```python
from build123d import *

# Parameters (mm, degrees)
SKETCH041_R   = 1.6
SKETCH041_R_2 = 5.98
PAD_DEPTH     = 5


with BuildPart() as part:
    # Sketch041 → Pad (new body)
    with BuildSketch(Plane.XZ):
        with BuildLine():
            Line((75.17, -33), (80.83, -33))
            Line((80.83, -33), (88.709309, -17.413936))
            ThreePointArc((88.709309, -17.413936), (89.672868, -14.782831), (90, -12))
            Line((90, -12), (90, -4))
            ThreePointArc((90, -4), (86.485281, 4.485281), (78, 8))
            Line((78, 8), (31, 8))
            ThreePointArc((28, 11), (28.87868, 8.87868), (31, 8))
            ThreePointArc((28, 11), (27.707107, 11.707107), (27, 12))
            Line((27, 12), (-19, 12))
            ThreePointArc((-19, 12), (-19.707107, 11.707107), (-20, 11))
            Line((-20, 11), (-20, -24))
            Line((-20, -24), (72.36, -24))
            Line((72.36, -24), (75.17, -33))
        make_face()
        with Locations((-14, 7)):
            Circle(SKETCH041_R, mode=Mode.SUBTRACT)
        with Locations((-2, -18)):
            Circle(SKETCH041_R, mode=Mode.SUBTRACT)
        Circle(SKETCH041_R_2, mode=Mode.SUBTRACT)
        with Locations((78, -12)):
            Circle(SKETCH041_R_2, mode=Mode.SUBTRACT)
        with BuildLine():
            ThreePointArc((7.5, -12.2), (8.027208, -13.472792), (9.3, -14))
            Line((9.3, -14), (13.2, -14))
            ThreePointArc((13.2, -14), (14.472792, -13.472792), (15, -12.2))
            Line((15, -12.2), (15, -9.8))
            ThreePointArc((15, -9.8), (14.472792, -8.527208), (13.2, -8))
            Line((13.2, -8), (9.3, -8))
            ThreePointArc((9.3, -8), (8.027208, -8.527208), (7.5, -9.8))
            Line((7.5, -9.8), (7.5, -12.2))
        make_face(mode=Mode.SUBTRACT)
        with BuildLine():
            Line((17.7, -4.5), (24.3, -4.5))
            ThreePointArc((24.3, -4.5), (25.148528, -4.148528), (25.5, -3.3))
            Line((25.5, -3.3), (25.5, -2.7))
            ThreePointArc((25.5, -2.7), (25.148528, -1.851472), (24.3, -1.5))
            Line((24.3, -1.5), (17.7, -1.5))
            ThreePointArc((17.7, -1.5), (16.851472, -1.851472), (16.5, -2.7))
            Line((16.5, -2.7), (16.5, -3.3))
            ThreePointArc((16.5, -3.3), (16.851472, -4.148528), (17.7, -4.5))
        make_face(mode=Mode.SUBTRACT)
        with BuildLine():
            Line((17.7, -16), (24.3, -16))
            ThreePointArc((24.3, -16), (25.148528, -15.648528), (25.5, -14.8))
            Line((25.5, -14.8), (25.5, -12.2))
            ThreePointArc((25.5, -12.2), (25.148528, -11.351472), (24.3, -11))
            Line((24.3, -11), (17.7, -11))
            ThreePointArc((17.7, -11), (16.851472, -11.351472), (16.5, -12.2))
            Line((16.5, -12.2), (16.5, -14.8))
            ThreePointArc((16.5, -14.8), (16.851472, -15.648528), (17.7, -16))
        make_face(mode=Mode.SUBTRACT)
    extrude(amount=PAD_DEPTH)


solid = part.part
```
Geometry check sheet. Reference: the model listing, model coordinates, mm. A direction names the side the tool comes from. Round coordinates to 2 decimals unless told otherwise and drop trailing zeros. Order: outer loops, then holes, each group sorted by start corner. A loop starts at its lowest first (then second) coordinate and runs counter-clockwise, first axis right, second up. Notation, with made-up numbers: (51.5, -16) -> (96.5, -16) arc R16 cw to (96.5, -9) -> close; hole circle Ø11 at (39, 49.25). An arc over 180 degrees is marked (long way). Return JSON: item names as keys, results as strings. Group by question number.
Q1. Material ranges on probe 1 along Z at (x, y) = (78, -0.95); probe 2 along Z at (x, y) = (-14, -3.9); probe 3 along X at (y, z) = (-2.35, -2.5), recorded low to high. Write a range as from..to.
Q2. Gauge pin test, flat ends, axial feed: pin 1 (3 mm diameter, centred on y = -2.5, z = -13.5, fed in from +X); pin 2 (2.5 mm diameter, centred on x = 20.5, y = -3.5, fed in from -Z); pin 3 (2.5 mm diameter, centred on x = 51.5, y = -3, fed in from +Z); pin 4 (1 mm diameter, centred on y = -2.5, z = -27.5, fed in from +X). Record the tip position at first contact, or that the pin passes through.
Q3. Release check for a two-part mould opening along X. For faces 1 (the flat face through (55, -2, 8)), 2 (the flat face through (-20, -2, -6)), 3 (the flat face through (21, -2, -4.5)) record: released by +X, released by -X, zero draft, split by the parting line, or undercut.
Q4. Section check B-B, the plane x = -2. Record the boundary of the cut face in (y, z), plus the area to 3 significant figures.
Q5. Section check D-D, the plane x = 46. Record the boundary of the cut face in (y, z).
Q6. Section check A-A, the plane z = 7. Record the boundary of the cut face in (x, y).
Q7. Section check C-C, the plane y = -1.25. Count the separate pieces of the cut face and the enclosed holes in it, plus the area to 3 significant figures.
Q8. Tool access check on faces 4 (the flat face through (26, -2, -24)), 5 (the cylindrical face through (28.86, -2.46, 8.9)), 6 (the flat face through (25.5, -2, -14)). Record the directions out of +Z, -Z, +X, -X, +Y, -Y that give a thin tool (end or side, any length) a straight path to the whole face; none if there is none.
Numbers:
{
 "1": {"probe 1": "-33..-17.98, -6.02..8", "probe 2": "-24..5.4, 8.6..12", "probe 3": "-20..-5.43, 5.43..16.52, 25.48..89.91"},
 "2": {"pin 1": "x = 90", "pin 2": "z = -24", "pin 3": "z = 8", "pin 4": "x = 83.86"},
 "3": {"face 1": "zero draft", "face 2": "released by -X", "face 3": "undercut"},
 "4": {"outline": "(-5, -24) -> (0, -24) -> (0, -19.6) -> (-5, -19.6) -> close; (-5, -16.4) -> (0, -16.4) -> (0, -5.64) -> (-5, -5.64) -> close; (-5, 5.64) -> (0, 5.64) -> (0, 12) -> (-5, 12) -> close", "area": "108 mm^2"},
 "5": {"outline": "(-5, -24) -> (0, -24) -> (0, 8) -> (-5, 8) -> close"},
 "6": {"outline": "(-20, -5) -> (-15.6, -5) -> (-15.6, 0) -> (-20, 0) -> close; (-12.4, -5) -> (82.8, -5) -> (82.8, 0) -> (-12.4, 0) -> close"},
 "7": {"separate pieces": "1", "enclosed holes": "7", "area": "3,390 mm^2"},
 "8": {"face 4": "-Z, -X, +Y, -Y", "face 5": "+Z, +X, +Y, -Y", "face 6": "+Y, -Y"}
}
